Source: CAD feature listing. Evaluate the final solid. Frame: model axes, mm. A direction names the side the tool comes from. Round coordinates to 2 decimals unless told otherwise and drop trailing zeros. Order: outer loops, then holes, each group sorted by start corner. A loop starts at its lowest first (then second) coordinate and runs counter-clockwise, first axis right, second up. Notation, with made-up numbers: (51, 86) -> (61, 86) arc R23 ccw to (61, 122) -> close; hole circle Ø10 at (82, -25.75). An arc over 180 degrees is marked (long way). Use a Markdown table: item, result. Add a question column.
```python
from build123d import *

# Parameters (mm, degrees)
F0_W        = 88.8999994576
F0_H        = 95.6510528922
F1_DEPTH    = 6.35
F2_DEPTH    = 25.4
F3_DEPTH    = 50.8
F4_R        = 6.34999
F5_SIZE2    = 7.3323484187
F5_SIZE     = 12.7
F6_C1_SIZE2 = 12.7
F6_C1_SIZE  = 7.3323484187
F6_C2_SIZE2 = 7.3323484187
F6_C2_SIZE  = 12.7
F6_C3_SIZE2 = 12.7
F6_C3_SIZE  = 7.3323484187
F6_C4_SIZE2 = 7.3323484187
F6_C4_SIZE  = 12.7


# Not quite as in the source:
# - a fillet or chamfer is up to 0.001 mm smaller than in the source, because OpenCascade refuses the exact size


with BuildPart() as f1:
    # F0 (on Top) → F1 (new body)
    with BuildSketch(Plane.XY):
        Rectangle(F0_W, F0_H)
        Polygon((-2.712e-07, 41.4755269885), (38.0999997288, 41.4755269885), (38.0999997288, 2.9744735539), (38.0999997288, -41.4755264461), (-2.712e-07, -41.4755264461), (-38.1000002712, -41.4755264461), (-38.1000002712, -2.9744730115), (-38.1000002712, 41.4755269885), align=None, mode=Mode.SUBTRACT)
    extrude(amount=F1_DEPTH)

    # F0 (on Top) → F2 (join)
    with BuildSketch(Plane.XY):
        with BuildLine():
            Line((38.0999997288, 2.9744735539), (38.0999997288, 41.4755269885))
            Line((38.0999997288, 41.4755269885), (-2.712e-07, 41.4755269885))
            Line((-2.712e-07, 41.4755269885), (-2.712e-07, 9.7255269885))
            ThreePointArc((-2.712e-07, 9.7255269885), (-3.7197441501, 0.7452708674), (-12.7000002712, -2.9744730115))
            Line((-12.7000002712, -2.9744730115), (-38.1000002712, -2.9744730115))
            Line((-38.1000002712, -2.9744730115), (-38.1000002712, -41.4755264461))
            Line((-38.1000002712, -41.4755264461), (-2.712e-07, -41.4755264461))
            Line((-2.712e-07, -41.4755264461), (-2.712e-07, -9.7255264461))
            ThreePointArc((-2.712e-07, -9.7255264461), (3.7197436077, -0.745270325), (12.6999997288, 2.9744735539))
            Line((12.6999997288, 2.9744735539), (38.0999997288, 2.9744735539))
        make_face()
    extrude(amount=F2_DEPTH)

    # F0 (on Top) → F3 (join)
    with BuildSketch(Plane.XY):
        with BuildLine():
            Line((-2.712e-07, 9.7255269885), (-2.712e-07, 41.4755269885))
            Line((-2.712e-07, 41.4755269885), (-38.1000002712, 41.4755269885))
            Line((-38.1000002712, 41.4755269885), (-38.1000002712, -2.9744730115))
            Line((-38.1000002712, -2.9744730115), (-12.7000002712, -2.9744730115))
            ThreePointArc((-12.7000002712, -2.9744730115), (-3.7197441501, 0.7452708674), (-2.712e-07, 9.7255269885))
        make_face()
        with BuildLine():
            Line((38.0999997288, -41.4755264461), (38.0999997288, 2.9744735539))
            Line((38.0999997288, 2.9744735539), (12.6999997288, 2.9744735539))
            ThreePointArc((12.6999997288, 2.9744735539), (3.7197436077, -0.745270325), (-2.712e-07, -9.7255264461))
            Line((-2.712e-07, -9.7255264461), (-2.712e-07, -41.4755264461))
            Line((-2.712e-07, -41.4755264461), (38.0999997288, -41.4755264461))
        make_face()
    extrude(amount=F3_DEPTH)

    # F4 (radius 6.35 in the source; OpenCascade refuses exactly that, so slightly less here)
    f4_edges = [f1.edges().sort_by_distance(p)[0] for p in [
        (44.45, 0, 6.35),
        (0, -47.825526, 6.35),
        (0, 47.825526, 6.35),
        (-44.45, 0, 6.35),
    ]]
    fillet(f4_edges, radius=F4_R)

    # F5
    f5_edges = [f1.edges().sort_by_distance(p)[0] for p in [
        (38.1, 22.225, 25.4),
        (19.05, 41.475527, 25.4),
        (-38.1, -22.225, 25.4),
        (-19.05, -41.475526, 25.4),
    ]]
    chamfer(f5_edges, length=F5_SIZE, length2=F5_SIZE2)

    # F6: chamfer of 12.7 x 7.3323484187 on 4 edges, made by hand

    # F6_c1
    f6_c1_edges = [f1.edges().sort_by_distance(p)[0] for p in [
        (-19.0500002712, 41.4755269885, 50.8),
    ]]
    f6_c1_side = f1.faces().sort_by_distance((-19.0500002712, 41.4755269885, 50.6533530316))[0]
    chamfer(f6_c1_edges, length=F6_C1_SIZE, length2=F6_C1_SIZE2, reference=f6_c1_side)

    # F6_c2
    f6_c2_edges = [f1.edges().sort_by_distance(p)[0] for p in [
        (38.0999997288, -19.2505264461, 50.8),
    ]]
    f6_c2_side = f1.faces().sort_by_distance((38.0999997288, -19.2505264461, 50.6533530316))[0]
    chamfer(f6_c2_edges, length=F6_C2_SIZE, length2=F6_C2_SIZE2, reference=f6_c2_side)

    # F6_c3
    f6_c3_edges = [f1.edges().sort_by_distance(p)[0] for p in [
        (-38.1000002712, 12.9005269885, 50.8),
    ]]
    f6_c3_side = f1.faces().sort_by_distance((-38.1000002712, 12.9005269885, 50.6533530316))[0]
    chamfer(f6_c3_edges, length=F6_C3_SIZE, length2=F6_C3_SIZE2, reference=f6_c3_side)

    # F6_c4
    f6_c4_edges = [f1.edges().sort_by_distance(p)[0] for p in [
        (15.3838255194, -41.4755264461, 50.8),
    ]]
    f6_c4_side = f1.faces().sort_by_distance((15.3838255194, -41.4755264461, 50.6533530316))[0]
    chamfer(f6_c4_edges, length=F6_C4_SIZE, length2=F6_C4_SIZE2, reference=f6_c4_side)


solid = f1.part
```
1) Section D-D on z = 41. Output: boundary loops of the cut face in (x, y).
2) First-contact query: pin 1 Ø12 at (x, y) = (-18.5, -18.5) entering from +Z; pin 2 Ø20.5 at (x, z) = (-22.5, 33.5) entering from -Y; pin 3 Ø18.5 at (y, z) = (9, 32.5) entering from -X. Flat tips, straight axial feed; report the tip coordinate or a pass-through.
3) Line query: probe 1 along Z at (x, y) = (25, 42); probe 2 along X at (y, z) = (-35, 29.5); probe 3 along Y at (x, z) = (24, 29.5). Output: solid intervals per line, ascending. Write a range as from..to.
4) Section A-A on z = 31.5. Output: boundary loops of the cut face in (x, y), then the cut area to 3 significant figures.
5) Reachability of faces 1 (the flat face through (0, 0, 25.4)), 2 (the flat face through (19.317, 37.758, 19.139)), 3 (the flat face through (-38.1, 10, 21)), 4 (the flat face through (38.1, -10, 18)) from +Z, -Z, +X, -X, +Y, -Y: full face, straight path, thin tool, end or side. Return the list, or none.
Conclusion:
| question | item | result |
|---|---|---|
| 1 | outline | (-38.1, -2.97) -> (-12.7, -2.97) arc R12.7 ccw to (0, 9.73) -> (0, 41.48) -> (-38.1, 41.48) -> close; (0, -39.8) -> (36.43, -39.8) -> (36.43, 2.97) -> (12.7, 2.97) arc R12.7 ccw to (0, -9.73) -> close |
| 2 | pin 1 | stops at z = 25.4 |
| 2 | pin 2 | stops at y = -35.38 |
| 2 | pin 3 | stops at x = -38.1 |
| 3 | probe 1 | z = 0..6.33 |
| 3 | probe 2 | x = 0..38.1 |
| 3 | probe 3 | y = -41.48..2.97 |
| 4 | outline | (-38.1, -2.97) -> (-12.7, -2.97) arc R12.7 ccw to (0, 9.73) -> (0, 41.48) -> (-38.1, 41.48) -> close; (0, -41.48) -> (38.1, -41.48) -> (38.1, 2.97) -> (12.7, 2.97) arc R12.7 ccw to (0, -9.73) -> close |
| 4 | area | 3,320 mm^2 |
| 5 | face 1 | +Z |
| 5 | face 2 | +Z, +X, +Y |
| 5 | face 3 | +Z, -X, +Y, -Y |
| 5 | face 4 | +Z, +X, +Y, -Y |
